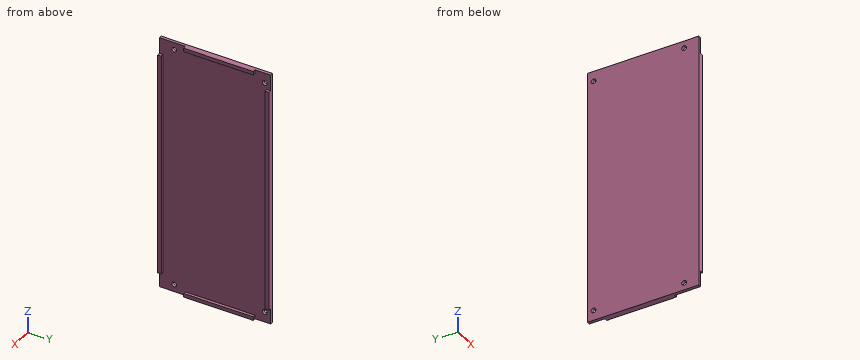
from build123d import *

# Parameters (mm, degrees)
SKETCH1_W           = 176
SKETCH1_H           = 75
SKETCH1_R           = 1.6
BOSS_EXTRUDE1_DEPTH = 2
SKETCH3_W           = 154
SKETCH3_H           = 2.5
BOSS_EXTRUDE2_DEPTH = 2
SKETCH4_W           = 2.5
SKETCH4_H           = 47
BOSS_EXTRUDE3_DEPTH = 2


with BuildPart() as part:
    # Sketch1 → Boss-Extrude1 (new body)
    with BuildSketch(Plane(origin=(0, 0, 0), x_dir=(0, 0, -1), z_dir=(1, 0, 0))):
        Rectangle(SKETCH1_W, SKETCH1_H)
        with Locations((-81, 33.5)):
            Circle(SKETCH1_R, mode=Mode.SUBTRACT)
        with Locations((81, 33.5)):
            Circle(SKETCH1_R, mode=Mode.SUBTRACT)
        with Locations((-83, -27.5)):
            Circle(SKETCH1_R, mode=Mode.SUBTRACT)
        with Locations((83, -27.5)):
            Circle(SKETCH1_R, mode=Mode.SUBTRACT)
    extrude(amount=BOSS_EXTRUDE1_DEPTH)

    # Sketch3 → Boss-Extrude2 (add)
    with BuildSketch(Plane(origin=(2, 0, 0), x_dir=(0, 0, -1), z_dir=(1, 0, 0))):
        with Locations((0, -36.25)):
            Rectangle(SKETCH3_W, SKETCH3_H)
        with Locations((0, 36.25)):
            Rectangle(SKETCH3_W, SKETCH3_H)
    extrude(amount=BOSS_EXTRUDE2_DEPTH)

    # Sketch4 → Boss-Extrude3 (add)
    with BuildSketch(Plane(origin=(2, 0, 0), x_dir=(0, 0, -1), z_dir=(1, 0, 0))):
        with Locations((-86.75, 3.5)):
            Rectangle(SKETCH4_W, SKETCH4_H)
        with Locations((86.75, 3.5)):
            Rectangle(SKETCH4_W, SKETCH4_H)
    extrude(amount=BOSS_EXTRUDE3_DEPTH)


solid = part.part
Work out the finished part from the listing and answer in its coordinate system (mm). Coordinates: 2 decimals unless noted, no trailing zeros. Loops run counter-clockwise (first coordinate to the right, second up) from the corner with the lowest first, then second, coordinate; pieces in that order, holes last. Notation, with made-up numbers: M 20,43.25 L 33,43.25 A14 ccw 33,63.25 Z; hole C 45,-5.5 d10. An arc over 180 degrees is marked long. Answer in a Markdown table with one row per item. Add a question column.
1. Find section B-B, the plane y = -27.5. Write down the section's boundary in (x, z), then the cut area to 3 significant figures.
2. Flat-ended cylindrical pins translate along their axes: P1, Ø0.6, axis at x = 2.5, z = -86.5, coming from the +Y side; P2, Ø5, axis at y = 2, z = 9.5, coming from the +X side; P3, Ø2, axis at x = 3.5, z = 87.5, coming from the -Y side. Find the tip coordinate at first contact, or state that the pin passes through.
3. Find section D-D, the plane z = 33.5. Write down the section's boundary in (x, y).
4. Find section A-A, the plane x = 2.9. Write down the section's boundary in (y, z), then the cut area to 4 significant figures.
5. Find section C-C, the plane y = -11. Write down the section's boundary in (x, z).
6. Consider L1, parallel to Z at x = 2.25, y = -2; L2, parallel to Y at x = 1.5, z = -83; L3, parallel to Y at x = 3.45, z = 37. Determine where each line is inside the solid, lowest interval first.
Reported:
| question | item | result |
|---|---|---|
| 1 | outline | M 0,-88 L 2,-88 L 2,-84.6 L 0,-84.6 Z; M 0,-81.4 L 2,-81.4 L 2,81.4 L 0,81.4 Z; M 0,84.6 L 2,84.6 L 2,88 L 0,88 Z |
| 1 | area | 339 mm^2 |
| 2 | P1 | stops at y = 27 |
| 2 | P2 | stops at x = 2 |
| 2 | P3 | stops at y = -20 |
| 3 | outline | M 0,-37.5 L 4,-37.5 L 4,-35 L 2,-35 L 2,35 L 4,35 L 4,37.5 L 0,37.5 Z |
| 4 | outline | M -37.5,-77 L -35,-77 L -35,77 L -37.5,77 Z; M -20,-88 L 27,-88 L 27,-85.5 L -20,-85.5 Z; M -20,85.5 L 27,85.5 L 27,88 L -20,88 Z; M 35,-77 L 37.5,-77 L 37.5,77 L 35,77 Z |
| 4 | area | 1,005 mm^2 |
| 5 | outline | M 0,-88 L 4,-88 L 4,-85.5 L 2,-85.5 L 2,85.5 L 4,85.5 L 4,88 L 0,88 Z |
| 6 | L1 | z = -88 to -85.5, 85.5 to 88 |
| 6 | L2 | y = -37.5 to -29.1, -25.9 to 37.5 |
| 6 | L3 | y = -37.5 to -35, 35 to 37.5 |
